```python
from build123d import *

# Parameters (mm, degrees)
SKETCH1_R           = 4.7625
BOSS_EXTRUDE1_DEPTH = 101.6
SKETCH2_W           = 11.315378495
SKETCH2_H           = 2.135355531
CUT_EXTRUDE1_DEPTH  = 19.05
SKETCH3_W           = 2.441021898
SKETCH3_H           = 8.016208274
CUT_EXTRUDE2_DEPTH  = 19.05
FILLET1_R           = 2.54
SKETCH4_R           = 4.572
BOSS_EXTRUDE2_DEPTH = 25.4
FILLET2_R           = 2.54


with BuildPart() as part:
    # Sketch1 → Boss-Extrude1 (new body)
    with BuildSketch(Plane(origin=(0, 0, 0), x_dir=(1, 0, 0), z_dir=(0, 1, 0))):
        with Locations(Location((0, 0, 0), (0, 0, 270))):
            Circle(SKETCH1_R)
    extrude(amount=-BOSS_EXTRUDE1_DEPTH)

    # Sketch2 → Cut-Extrude1 (cut)
    with BuildSketch(Plane(origin=(0, 0, 0), x_dir=(1, 0, 0), z_dir=(0, 1, 0))):
        with Locations((0.38675801, 4.877677766)):
            Rectangle(SKETCH2_W, SKETCH2_H)
        with Locations((-0.38675801, -4.877677766)):
            Rectangle(SKETCH2_W, SKETCH2_H)
    extrude(amount=-CUT_EXTRUDE1_DEPTH, mode=Mode.SUBTRACT)

    # Sketch3 → Cut-Extrude2 (cut)
    with BuildSketch(Plane(origin=(0, 0, 0), x_dir=(1, 0, 0), z_dir=(0, 1, 0))):
        with Locations((5.030510949, -0.198104137)):
            Rectangle(SKETCH3_W, SKETCH3_H)
        with Locations((-5.030510949, 0.198104137)):
            Rectangle(SKETCH3_W, SKETCH3_H)
    extrude(amount=-CUT_EXTRUDE2_DEPTH, mode=Mode.SUBTRACT)

    # Fillet1
    # the kernel refuses this fillet: 2.54 mm, written as the material it adds along each edge
    with BuildSketch(Plane(origin=(9.2075, -19.05, -3.81), x_dir=(0, 1, 0), z_dir=(-1, 0, 0))) as fillet1_piece_1_section:
        with BuildLine():
            CenterArc((FILLET1_R, FILLET1_R), FILLET1_R, 180, 90)
            Line((0, FILLET1_R), (0, 0))
            Line((0, 0), (FILLET1_R, 0))
        make_face()
    fillet1_piece_1 = extrude(amount=18.415, mode=Mode.PRIVATE)
    fillet1_piece_1 = fillet1_piece_1 & Plane(origin=(0, -18.276812149, 0), x_dir=(0, 0, 1), z_dir=(0, 1, 0)) * Cylinder(4.7625, 47, mode=Mode.PRIVATE)
    add(fillet1_piece_1)
    with BuildSketch(Plane(origin=(3.81, -19.05, 9.2075), x_dir=(0, 1, 0), z_dir=(0, 0, -1))) as fillet1_piece_2_section:
        with BuildLine():
            CenterArc((FILLET1_R, FILLET1_R), FILLET1_R, 180, 90)
            Line((0, FILLET1_R), (0, 0))
            Line((0, 0), (FILLET1_R, 0))
        make_face()
    fillet1_piece_2 = extrude(amount=18.415, mode=Mode.PRIVATE)
    fillet1_piece_2 = fillet1_piece_2 & Plane(origin=(0, -18.276812149, 0), x_dir=(0, 0, 1), z_dir=(0, 1, 0)) * Cylinder(4.7625, 47, mode=Mode.PRIVATE)
    add(fillet1_piece_2)
    with BuildSketch(Plane(origin=(-3.81, -19.05, -9.2075), x_dir=(0, 1, 0), z_dir=(0, 0, 1))) as fillet1_piece_3_section:
        with BuildLine():
            CenterArc((FILLET1_R, FILLET1_R), FILLET1_R, 180, 90)
            Line((0, FILLET1_R), (0, 0))
            Line((0, 0), (FILLET1_R, 0))
        make_face()
    fillet1_piece_3 = extrude(amount=18.415, mode=Mode.PRIVATE)
    fillet1_piece_3 = fillet1_piece_3 & Plane(origin=(0, -18.276812149, 0), x_dir=(0, 0, 1), z_dir=(0, 1, 0)) * Cylinder(4.7625, 47, mode=Mode.PRIVATE)
    add(fillet1_piece_3)
    with BuildSketch(Plane(origin=(9.2075, -19.05, 3.81), x_dir=(0, 0, 1), z_dir=(-1, 0, 0))) as fillet1_piece_4_section:
        with BuildLine():
            CenterArc((FILLET1_R, FILLET1_R), FILLET1_R, 180, 90)
            Line((0, FILLET1_R), (0, 0))
            Line((0, 0), (FILLET1_R, 0))
        make_face()
    fillet1_piece_4 = extrude(amount=18.415, mode=Mode.PRIVATE)
    fillet1_piece_4 = fillet1_piece_4 & Plane(origin=(0, -18.276814904, 0), x_dir=(0, 0, 1), z_dir=(0, 1, 0)) * Cylinder(4.7625, 47, mode=Mode.PRIVATE)
    add(fillet1_piece_4)

    # Sketch4 → Boss-Extrude2 (add)
    with BuildSketch(Plane.XZ.offset(101.6)):
        with Locations(Location((0, 0, 0), (0, 0, 270))):
            Circle(SKETCH4_R)
    extrude(amount=BOSS_EXTRUDE2_DEPTH)

    # Fillet2
    # the kernel refuses this fillet: 2.54 mm, written as the material it adds along each edge
    with BuildSketch(Plane(origin=(0, -101.6, 0), x_dir=(0, 0, -1), z_dir=(-1, 0, 0))) as fillet2_piece_1:
        with BuildLine():
            CenterArc((7.112, 0.965116444), FILLET2_R, 180, 22.331645009)
            Line((4.572, 0.965116444), (4.5212, 0.965116444))
            Line((4.5212, 0.965116444), (4.5212, 0))
            Line((4.5212, 0), (4.572, -0.0508))
            ThreePointArc((4.572, -0.0508), (4.66725, -0.0508), (4.71551, -0.019302329))
            Line((4.71551, -0.019302329), (4.7625, 0))
        make_face()
    revolve(axis=Axis((0, -101.6, 0), (0, -1, 0)))


solid = part.part
```
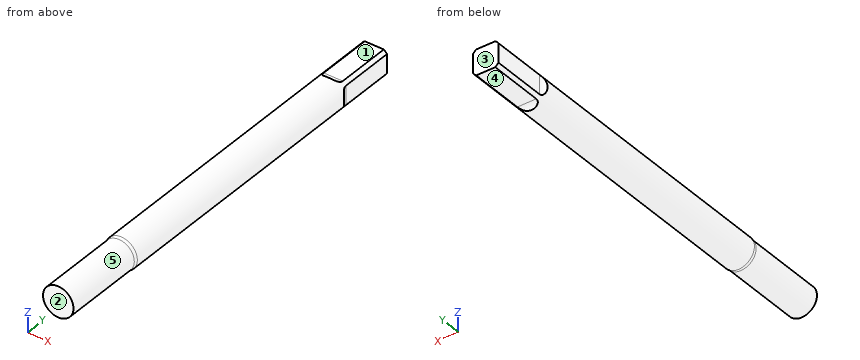
Verification items for the finished model (mm, model axes). Face numbers are marked on the shaded views. A direction names the side the tool comes from. Round coordinates to 2 decimals unless told otherwise and drop trailing zeros. Order: outer loops, then holes, each group sorted by start corner. A loop starts at its lowest first (then second) coordinate and runs counter-clockwise, first axis right, second up.
1) Tool access check on the marked faces 1, 2, 3, 4 and 5. Record the directions out of +Z, -Z, +X, -X, +Y, -Y that give a thin tool (end or side, any length) a straight path to the whole face; none if there is none.
Geometry says:
face 1: +Z, +X, -X, +Y
face 2: +Z, -Z, +X, -X, -Y
face 3: +Z, -Z, +X, -X, +Y
face 4: -Z, +X, -X, +Y
face 5: -Y
2) Cross-section at C-C, the plane y = -64.5. Record the cut outline in (x, z) (1 decimal).
Geometry says:
outline: circle Ø9.5 at (0, 0)
3) Cross-section at A-A, the plane z = 0. Record the cut outline in (x, y), plus the area to 3 significant figures.
Geometry says:
outline: (-4.76, -101.6) arc R2.54 cw to (-4.57, -102.57) - (-4.57, -127) - (4.57, -127) - (4.57, -102.57) arc R2.54 cw to (4.76, -101.6) - (4.76, -18.49) arc R2.54 cw to (3.81, -16.51) - (3.81, 0) - (-3.81, 0) - (-3.81, -16.51) arc R2.54 cw to (-4.76, -18.49) - close
area: 1,170 mm2
4) Material ranges on line 1 (Z direction, x = -0.25, y = -110.5); line 2 (X direction, y = -15.5, z = 0.25); line 3 (Z direction, x = -1.75, y = -38), recorded low to high.
Geometry says:
line 1: z = -4.57 to 4.57
line 2: x = -3.81 to 3.81
line 3: z = -4.43 to 4.43
5) Depth check by flat-ended pin: pin 1 (3 mm diameter, centred on y = -10.5, z = -1, fed in from -X); pin 2 (4.5 mm diameter, centred on y = -6.5, z = -1.5, fed in from +X); pin 3 (1 mm diameter, centred on y = -59.5, z = -2, fed in from +X). Enter the tip coordinate at first touch or a pass-through.
Geometry says:
pin 1: stops at x = -3.81
pin 2: stops at x = 3.81
pin 3: stops at x = 4.52
6) Cross-section at B-B, the plane x = 0. Record the cut outline in (y, z), plus the area to 3 significant figures.
Geometry says:
outline: (-127, -4.57) - (-102.57, -4.57) arc R2.54 cw to (-101.6, -4.76) - (-18.49, -4.76) arc R2.54 cw to (-16.51, -3.81) - (0, -3.81) - (0, 3.81) - (-16.51, 3.81) arc R2.54 cw to (-18.49, 4.76) - (-101.6, 4.76) arc R2.54 cw to (-102.57, 4.57) - (-127, 4.57) - close
area: 1,170 mm2
